from build123d import *

# Parameters (mm, degrees)
EXTRUDE_1_DEPTH             = 7.5
HOLE_WIZARD_M51_D           = 5.5
HOLE_WIZARD_M51_CSINK_D     = 10.4
HOLE_WIZARD_M51_CSINK_ANGLE = 90


with BuildPart() as part:
    # Эскиз1 → Бобышка-Вытянуть1 (new, symmetric)
    with BuildSketch(Plane.XY):
        Polygon((-10, 0), (-10, 10), (10, 10), (10, 0), (16, 0), (29.505188455, 57.41043399), (27.505188455, 57.41043399), (10, 32.41043399), (-10, 32.41043399), (-27.505188455, 57.41043399), (-29.505188455, 57.41043399), (-16, 0), align=None)
    extrude(amount=EXTRUDE_1_DEPTH, both=True)

    # Зенковка для  винта с плоской головкой M51 (through all)
    with Locations(Plane.ZX.offset(32.41043399)):
        with Locations((0, 0)):
            CounterSinkHole(HOLE_WIZARD_M51_D / 2, HOLE_WIZARD_M51_CSINK_D / 2, counter_sink_angle=HOLE_WIZARD_M51_CSINK_ANGLE)


solid = part.part
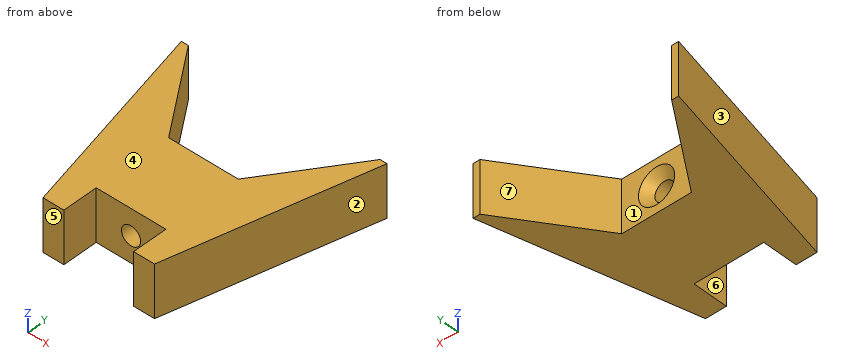
Verification items for the finished model (mm, model axes). Face numbers are marked on the shaded views. A direction names the side the tool comes from. Coordinates: 2 decimals unless noted, no trailing zeros. Order: outer loops, then holes, each group sorted by start corner. A loop starts at its lowest first (then second) coordinate and runs counter-clockwise, first axis right, second up. Notation, with made-up numbers: M 29.5,30 L 46.5,30 A29 cw 46.5,57 Z; hole C 53.5,74.25 d3. An arc over 180 degrees is marked long. One line per item, written item: value. Start each with the question number.
Item 1: Mould release check, pull along X, two halves, no side actions. Record for the marked faces 1, 2, 3 and 4: released by +X, released by -X, zero draft, split by the parting line, or undercut.
Item 2: Gauge pin test, flat ends, axial feed: pin 1 (2 mm diameter, centred on x = 18, z = 0.5, fed in from +Y); pin 2 (6 mm diameter, centred on y = 15, z = 3, fed in from -X); pin 3 (1.5 mm diameter, centred on x = 9.5, z = 2.5, fed in from +Y). Record the tip position at first contact, or that the pin passes through.
Item 3: Access from +Z, -Z, +X, -X, +Y, -Y to the whole of each face (thin tool, end or side, straight path). Record for the marked faces 5, 6 and 7.
Item 4: Sectioned sample at B-B (z = 0). Enter the section's corners in (x, y).
Item 5: Scan lines: probe 1 along Z at (x, y) = (0, 25); probe 2 along X at (y, z) = (35.5, 0); probe 3 along Y at (x, z) = (-1, 6). Record each from-to range of solid material in increasing order.
Item 6: Sectioned sample at D-D (x = -8). Enter the section's corners in (y, z).
Item 7: Sectioned sample at C-C (y = 22). Enter the section's corners in (x, z), then the cut area to 4 significant figures.
Item 8: Sectioned sample at A-A (x = 0). Enter the section's corners in (y, z).
Conclusion:
1. face 1: undercut
1. face 2: released by +X
1. face 3: released by -X
1. face 4: zero draft
2. pin 1: stops at y = 45.26
2. pin 2: stops at x = -20.23
2. pin 3: stops at y = 32.77
3. face 5: +Z, -Z, +X, -X, -Y
3. face 6: +Z, -Z, -Y
3. face 7: +Z, -Z, +Y
4. outline: M -29.51,57.41 L -16,0 L -10,0 L -10,10 L -2.75,10 L -2.75,29.96 L -5.2,32.41 L -10,32.41 L -27.51,57.41 Z; M 2.75,10 L 10,10 L 10,0 L 16,0 L 29.51,57.41 L 27.51,57.41 L 10,32.41 L 5.2,32.41 L 2.75,29.96 Z
5. probe 1: z = -7.5 to -2.75, 2.75 to 7.5
5. probe 2: x = -24.35 to -12.16, 12.16 to 24.35
5. probe 3: y = 10 to 32.41
6. outline: M 10,-7.5 L 32.41,-7.5 L 32.41,7.5 L 10,7.5 Z
7. outline: M -21.18,-7.5 L 21.18,-7.5 L 21.18,7.5 L -21.18,7.5 Z; hole C 0,0 d5.5
7. area: 611.5 mm^2
8. outline: M 10,-7.5 L 32.41,-7.5 L 32.41,-5.2 L 29.96,-2.75 L 10,-2.75 Z; M 10,2.75 L 29.96,2.75 L 32.41,5.2 L 32.41,7.5 L 10,7.5 Z
